from build123d import *

# Parameters (mm, degrees)
BOSS_EXTRUDE1_DEPTH                 = 170
CUT_EXTRUDE2_DEPTH                  = 1378.200029658
CUT_EXTRUDE2_DEPTH_BACK             = 1378.200029658
SKETCH7_W                           = 60.055026026
SKETCH7_H                           = 40
SKETCH7_H_2                         = 30
CUT_EXTRUDE7_DEPTH                  = 20.697901
FILLET1_R                           = 10
CUT_EXTRUDE3_REACH                  = 1001.772
CUT_EXTRUDE3_END_RADIUS             = 68.41639524
SKETCH3_R                           = 2.5
CUT_EXTRUDE3_DIRECTION_2_DEPTH      = 10
SKETCH4_R                           = 2.5
CUT_EXTRUDE4_DEPTH                  = 10
CUT_EXTRUDE4_DIRECTION_2_REACH      = 1377.394
CUT_EXTRUDE4_DIRECTION_2_END_RADIUS = 68.41639524
CUT_EXTRUDE5_REACH                  = 1377.394
SKETCH5_R                           = 5
CUT_EXTRUDE6_REACH                  = 1001.772
SKETCH6_R                           = 5


with BuildPart() as part:
    # Sketch1 → Boss-Extrude1 (new body)
    with BuildSketch(Plane.XY):
        with BuildLine():
            Line((1349.709167159, 7.051545827), (1340.728911037, -1.928710294))
            Line((1340.728911037, -1.928710294), (1340.375357647, -2.282263684))
            Line((1340.375357647, -2.282263684), (1361.562180969, -23.469087006))
            Line((1361.562180969, -23.469087006), (1354.491113157, -30.540154818))
            ThreePointArc((1354.491113157, -30.540154818), (1332.276376869, -15.701535719), (1306.072590331, -10.501468778))
            Line((1306.072590331, -10.501468778), (1306.072590331, -0.501468778))
            Line((1306.072590331, -0.501468778), (1336.035283217, -0.501468778))
            Line((1336.035283217, -0.501468778), (1336.035283217, -0.001468778))
            Line((1336.035283217, -0.001468778), (1336.072590331, 12.698531222))
            Line((1336.072590331, 12.698531222), (1336.072590331, 13.198531222))
            Line((1336.072590331, 13.198531222), (1321.072590331, 13.198531222))
            Line((1321.072590331, 13.198531222), (1321.072590331, 21.198531222))
            ThreePointArc((1321.072590331, 21.198531222), (1345.563373492, 16.327364444), (1366.326176516, 2.45535175))
            Line((1366.326176516, 2.45535175), (1360.669322267, -3.2015025))
            Line((1360.669322267, -3.2015025), (1350.062720549, 7.405099218))
            Line((1350.062720549, 7.405099218), (1349.709167159, 7.051545827))
        make_face()
    extrude(amount=-BOSS_EXTRUDE1_DEPTH)

    # Sketch2 → Cut-Extrude2 (cut, two sides: drawn at the far end of the back side and taken through both)
    with BuildSketch(Plane(origin=(0, 0, 0), x_dir=(1, 0, 0), z_dir=(0, 1, 0)).offset(-CUT_EXTRUDE2_DEPTH_BACK)):
        Polygon((1306.072590331, 165.353911181), (1366.326176516, 140.977580956), (1366.326176516, 170), (1306.072590331, 170), align=None)
        Polygon((1366.326176516, 4.246407684), (1353.192629401, 0), (1366.326176516, 0), align=None)
    extrude(amount=CUT_EXTRUDE2_DEPTH + CUT_EXTRUDE2_DEPTH_BACK, mode=Mode.SUBTRACT)

    # Sketch7 → Cut-Extrude7 (cut)
    with BuildSketch(Plane(origin=(187.283823237, 452.52498352, 0), x_dir=(-0.923993669874315, 0.38240776408461624, 0), z_dir=(-0.3824077640846163, -0.9239936698743151, 0))):
        with Locations((-1237.02208443, 145.353911181)):
            Rectangle(SKETCH7_W, SKETCH7_H)
        with Locations((-1237.02208443, 15)):
            Rectangle(SKETCH7_W, SKETCH7_H_2)
    extrude(amount=-CUT_EXTRUDE7_DEPTH, mode=Mode.SUBTRACT)

    # Fillet1
    fillet1_edges = [part.edges().sort_by_distance(p)[0] for p in [
        (1363.497749392, -0.373075375, -3.331905717),
        (1321.072590331, 17.198531222, 0),
        (1363.497749392, -0.373075375, -142.121855977),
        (1321.072590331, 17.198531222, -159.285476478),
        (1306.072590331, -5.501468778, -30),
        (1306.072590331, -5.501468778, -125.353911181),
        (1358.026647063, -27.004620912, -125.353911181),
        (1358.026647063, -27.004620912, -30),
    ]]
    fillet(fillet1_edges, radius=FILLET1_R)

    # Cut-Extrude3: up to this cylinder (the profile starts outside it)
    cut_extrude3_end = Plane(origin=(1306.113416139, -78.917851837, -77.676956), z_dir=(0, 0, 1)) * Cylinder(CUT_EXTRUDE3_END_RADIUS, 2201.37679048, mode=Mode.PRIVATE)
    # Sketch3 → Cut-Extrude3 (cut, up to the surface)
    with BuildSketch(Plane(origin=(661.975479169, 661.975479169, 0), x_dir=(0, 0, 1), z_dir=(0.7071067811866074, 0.7071067811864877, 0)), mode=Mode.PRIVATE) as cut_extrude3_sk1:
        with Locations(Location((-77.676955591, 971.365001741, 0), (0, 0, 270))):
            Circle(SKETCH3_R)
    cut_extrude3_tool1 = extrude(cut_extrude3_sk1.sketch, amount=-CUT_EXTRUDE3_REACH, mode=Mode.PRIVATE) - cut_extrude3_end
    add(cut_extrude3_tool1.solids().sort_by_distance((1348.834259, -24.883301, -77.676956))[0], mode=Mode.SUBTRACT)
    # Sketch3 → Cut-Extrude3 (cut, up to the surface)
    with BuildSketch(Plane(origin=(661.975479169, 661.975479169, 0), x_dir=(0, 0, 1), z_dir=(0.7071067811866074, 0.7071067811864877, 0)), mode=Mode.PRIVATE) as cut_extrude3_sk2:
        with Locations(Location((-107.676955591, 971.365001741, 0), (0, 0, 270))):
            Circle(SKETCH3_R)
    cut_extrude3_tool2 = extrude(cut_extrude3_sk2.sketch, amount=-CUT_EXTRUDE3_REACH, mode=Mode.PRIVATE) - cut_extrude3_end
    add(cut_extrude3_tool2.solids().sort_by_distance((1348.834259, -24.883301, -107.676956))[0], mode=Mode.SUBTRACT)
    # Sketch3 → Cut-Extrude3 (cut, up to the surface)
    with BuildSketch(Plane(origin=(661.975479169, 661.975479169, 0), x_dir=(0, 0, 1), z_dir=(0.7071067811866074, 0.7071067811864877, 0)), mode=Mode.PRIVATE) as cut_extrude3_sk3:
        with Locations(Location((-47.676955591, 971.365001741, 0), (0, 0, 270))):
            Circle(SKETCH3_R)
    cut_extrude3_tool3 = extrude(cut_extrude3_sk3.sketch, amount=-CUT_EXTRUDE3_REACH, mode=Mode.PRIVATE) - cut_extrude3_end
    add(cut_extrude3_tool3.solids().sort_by_distance((1348.834259, -24.883301, -47.676956))[0], mode=Mode.SUBTRACT)

    # Sketch3 → Cut-Extrude3 direction 2 (cut)
    with BuildSketch(Plane(origin=(661.975479169, 661.975479169, 0), x_dir=(0, 0, 1), z_dir=(0.7071067811866074, 0.7071067811864877, 0))):
        with Locations(Location((-77.676955591, 971.365001741, 0), (0, 0, 270))):
            Circle(SKETCH3_R)
        with Locations(Location((-107.676955591, 971.365001741, 0), (0, 0, 270))):
            Circle(SKETCH3_R)
        with Locations(Location((-47.676955591, 971.365001741, 0), (0, 0, 270))):
            Circle(SKETCH3_R)
    extrude(amount=CUT_EXTRUDE3_DIRECTION_2_DEPTH, mode=Mode.SUBTRACT)

    # Sketch4 → Cut-Extrude4 (cut)
    with BuildSketch(Plane(origin=(0, -10.501468778, 0), x_dir=(0, 0, 1), z_dir=(0, -1, 0))):
        with Locations((-107.676955591, -1314.072590331)):
            Circle(SKETCH4_R)
        with Locations((-77.676955591, -1314.072590331)):
            Circle(SKETCH4_R)
        with Locations((-47.676955591, -1314.072590331)):
            Circle(SKETCH4_R)
    extrude(amount=-CUT_EXTRUDE4_DEPTH, mode=Mode.SUBTRACT)

    # Cut-Extrude4 direction 2: up to this cylinder (the profile starts outside it)
    cut_extrude4_direction_2_end = Plane(origin=(1306.113416139, -78.917851837, -77.676956), z_dir=(0, 0, 1)) * Cylinder(CUT_EXTRUDE4_DIRECTION_2_END_RADIUS, 2952.62079048, mode=Mode.PRIVATE)
    # Sketch4 → Cut-Extrude4 direction 2 (cut, up to the surface)
    with BuildSketch(Plane(origin=(0, -10.501468778, 0), x_dir=(0, 0, 1), z_dir=(0, -1, 0)), mode=Mode.PRIVATE) as cut_extrude4_direction_2_sk1:
        with Locations((-107.676955591, -1314.072590331)):
            Circle(SKETCH4_R)
    cut_extrude4_direction_2_tool1 = extrude(cut_extrude4_direction_2_sk1.sketch, amount=CUT_EXTRUDE4_DIRECTION_2_REACH, mode=Mode.PRIVATE) - cut_extrude4_direction_2_end
    add(cut_extrude4_direction_2_tool1.solids().sort_by_distance((1314.07259, -10.501469, -107.676956))[0], mode=Mode.SUBTRACT)
    # Sketch4 → Cut-Extrude4 direction 2 (cut, up to the surface)
    with BuildSketch(Plane(origin=(0, -10.501468778, 0), x_dir=(0, 0, 1), z_dir=(0, -1, 0)), mode=Mode.PRIVATE) as cut_extrude4_direction_2_sk2:
        with Locations((-77.676955591, -1314.072590331)):
            Circle(SKETCH4_R)
    cut_extrude4_direction_2_tool2 = extrude(cut_extrude4_direction_2_sk2.sketch, amount=CUT_EXTRUDE4_DIRECTION_2_REACH, mode=Mode.PRIVATE) - cut_extrude4_direction_2_end
    add(cut_extrude4_direction_2_tool2.solids().sort_by_distance((1314.07259, -10.501469, -77.676956))[0], mode=Mode.SUBTRACT)
    # Sketch4 → Cut-Extrude4 direction 2 (cut, up to the surface)
    with BuildSketch(Plane(origin=(0, -10.501468778, 0), x_dir=(0, 0, 1), z_dir=(0, -1, 0)), mode=Mode.PRIVATE) as cut_extrude4_direction_2_sk3:
        with Locations((-47.676955591, -1314.072590331)):
            Circle(SKETCH4_R)
    cut_extrude4_direction_2_tool3 = extrude(cut_extrude4_direction_2_sk3.sketch, amount=CUT_EXTRUDE4_DIRECTION_2_REACH, mode=Mode.PRIVATE) - cut_extrude4_direction_2_end
    add(cut_extrude4_direction_2_tool3.solids().sort_by_distance((1314.07259, -10.501469, -47.676956))[0], mode=Mode.SUBTRACT)

    # Sketch5 → Cut-Extrude5 (cut, up to next)
    with BuildSketch(Plane(origin=(0, -10.501468778, 0), x_dir=(0, 0, 1), z_dir=(0, -1, 0)), mode=Mode.PRIVATE) as cut_extrude5_sk1:
        with Locations((-47.676955591, -1314.072590331)):
            Circle(SKETCH5_R)
    cut_extrude5_tool1 = extrude(cut_extrude5_sk1.sketch, amount=CUT_EXTRUDE5_REACH, mode=Mode.PRIVATE) & part.part
    # Sketch5 → Cut-Extrude5 (cut, up to next)
    with BuildSketch(Plane(origin=(0, -10.501468778, 0), x_dir=(0, 0, 1), z_dir=(0, -1, 0)), mode=Mode.PRIVATE) as cut_extrude5_sk2:
        with Locations((-77.676955591, -1314.072590331)):
            Circle(SKETCH5_R)
    cut_extrude5_tool2 = extrude(cut_extrude5_sk2.sketch, amount=CUT_EXTRUDE5_REACH, mode=Mode.PRIVATE) & part.part
    # Sketch5 → Cut-Extrude5 (cut, up to next)
    with BuildSketch(Plane(origin=(0, -10.501468778, 0), x_dir=(0, 0, 1), z_dir=(0, -1, 0)), mode=Mode.PRIVATE) as cut_extrude5_sk3:
        with Locations((-107.676955591, -1314.072590331)):
            Circle(SKETCH5_R)
    cut_extrude5_tool3 = extrude(cut_extrude5_sk3.sketch, amount=CUT_EXTRUDE5_REACH, mode=Mode.PRIVATE) & part.part
    add(cut_extrude5_tool1.solids().sort_by_distance((1314.07259, -10.501469, -47.676956))[0], mode=Mode.SUBTRACT)
    add(cut_extrude5_tool2.solids().sort_by_distance((1314.07259, -10.501469, -77.676956))[0], mode=Mode.SUBTRACT)
    add(cut_extrude5_tool3.solids().sort_by_distance((1314.07259, -10.501469, -107.676956))[0], mode=Mode.SUBTRACT)

    # Sketch6 → Cut-Extrude6 (cut, up to next)
    with BuildSketch(Plane(origin=(661.975479169, 661.975479169, 0), x_dir=(0, 0, 1), z_dir=(0.7071067811866074, 0.7071067811864877, 0)), mode=Mode.PRIVATE) as cut_extrude6_sk1:
        with Locations(Location((-107.676955591, 971.365001741, 0), (0, 0, 270))):
            Circle(SKETCH6_R)
    cut_extrude6_tool1 = extrude(cut_extrude6_sk1.sketch, amount=-CUT_EXTRUDE6_REACH, mode=Mode.PRIVATE) & part.part
    # Sketch6 → Cut-Extrude6 (cut, up to next)
    with BuildSketch(Plane(origin=(661.975479169, 661.975479169, 0), x_dir=(0, 0, 1), z_dir=(0.7071067811866074, 0.7071067811864877, 0)), mode=Mode.PRIVATE) as cut_extrude6_sk2:
        with Locations(Location((-77.676955591, 971.365001741, 0), (0, 0, 270))):
            Circle(SKETCH6_R)
    cut_extrude6_tool2 = extrude(cut_extrude6_sk2.sketch, amount=-CUT_EXTRUDE6_REACH, mode=Mode.PRIVATE) & part.part
    # Sketch6 → Cut-Extrude6 (cut, up to next)
    with BuildSketch(Plane(origin=(661.975479169, 661.975479169, 0), x_dir=(0, 0, 1), z_dir=(0.7071067811866074, 0.7071067811864877, 0)), mode=Mode.PRIVATE) as cut_extrude6_sk3:
        with Locations(Location((-47.676955591, 971.365001741, 0), (0, 0, 270))):
            Circle(SKETCH6_R)
    cut_extrude6_tool3 = extrude(cut_extrude6_sk3.sketch, amount=-CUT_EXTRUDE6_REACH, mode=Mode.PRIVATE) & part.part
    add(cut_extrude6_tool1.solids().sort_by_distance((1348.834259, -24.883301, -107.676956))[0], mode=Mode.SUBTRACT)
    add(cut_extrude6_tool2.solids().sort_by_distance((1348.834259, -24.883301, -77.676956))[0], mode=Mode.SUBTRACT)
    add(cut_extrude6_tool3.solids().sort_by_distance((1348.834259, -24.883301, -47.676956))[0], mode=Mode.SUBTRACT)


solid = part.part
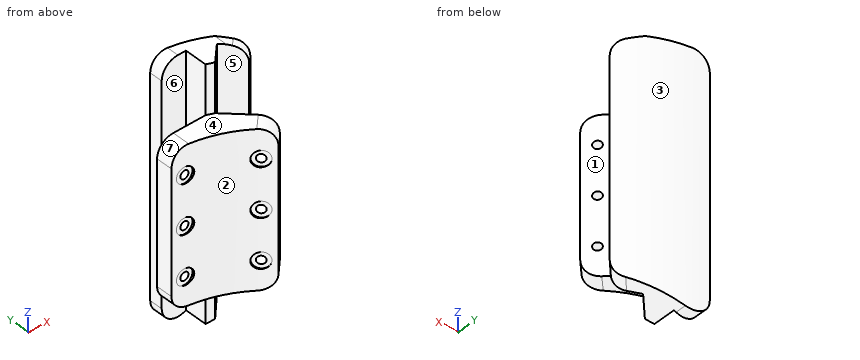
Can you work these out from the model? Positions are in its coordinate system, mm. Face numbers are marked on the shaded views. A direction names the side the tool comes from. Give positions to 0.01 mm unless a question says otherwise; leave off trailing zeros. Loops run counter-clockwise (first coordinate to the right, second up) from the corner with the lowest first, then second, coordinate; pieces in that order, holes last. Notation, with made-up numbers: (-35.75, 48) -> (-25.75, 48) arc R19 cw to (-25.75, 66) -> close; hole circle Ø7 at (-13, 44). An arc over 180 degrees is marked (long way). Write item = value, one per line.
1) Suppose I cut it at B-B on z = -86. Write out the boundary of the cut face in (x, y), then the cut area to 3 significant figures.
Check result:
outline = (1306.07, -10.5) arc R68.42 cw to (1354.49, -30.54) -> (1361.56, -23.47) -> (1340.38, -2.28) -> (1350.06, 7.41) -> (1360.67, -3.2) -> (1366.33, 2.46) arc R64 ccw to (1321.07, 21.2) -> (1321.07, 13.2) -> (1336.07, 13.2) -> (1336.07, 12.7) -> (1336.04, 0) -> (1336.04, -0.5) -> (1306.07, -0.5) -> close
area = 1,170 mm2
2) Suppose I cut it at C-C on y = 15.5. Write out the boundary of the cut face in (x, z).
Check result:
outline = (1321.07, -144.45) arc R10 ccw to (1334.82, -153.72) -> (1347.47, -148.61) -> (1347.47, 0) -> (1331.07, 0) arc R10 ccw to (1321.07, -10) -> close
3) I need wall thicknesses on L1, parallel to Z at x = 1313.5, y = -3.5; L2, parallel to Z at x = 1342.5, y = -18; L3, parallel to Z at x = 1345, y = -22. Which ranges of each line are inside material? Lowest first, please. Write a range as from..to.
Check result:
L1 = -125.02..-110.11, -105.24..-80.11, -75.24..-50.11, -45.24..-30.34
L2 = -125.35..-30
L3 = -125.35..-109.24, -106.12..-79.24, -76.12..-49.24, -46.12..-30
4) Will these pins go through, and if not, where does the flat tip stop? pin 1 (5 mm diameter, centred on y = 9, z = -120.5, fed in from +X); pin 2 (13 mm diameter, centred on x = 1314.07, z = -77.68, fed in from +Y); pin 3 (6 mm diameter, centred on y = 12, z = -102.5, fed in from +X); pin 4 (4.5 mm diameter, centred on x = 1314.07, z = -47.68, fed in from -Y).
Check result:
pin_1 = 1361.88
pin_2 = -0.5
pin_3 = 1358.66
pin_4 = through
5) Thinking about a two-plate mould opening in Y: for the marked faces 1, 2, 3 and 4, which applies, released by +Y, released by -Y, zero draft, split by the parting line, or undercut?
Check result:
face_1 = undercut
face_2 = released by -Y
face_3 = released by +Y
face_4 = zero draft
6) For the marked faces 5, 6 and 7, which set-ups out of +Z, -Z, +X, -X, +Y, -Y let a thin tool reach every point of the face, with its end or its side?
Check result:
face_5 = +Z, -Z
face_6 = +Z, -Z, -X
face_7 = +Z, -X, +Y, -Y
7) Suppose I cut it at A-A on x = 1328. Write out the boundary of the cut face in (y, z).
Check result:
outline = (-14.1, -125.35) -> (-0.5, -125.35) -> (-0.5, -30) -> (-14.1, -30) -> close; (13.2, -153.97) -> (20.82, -153.97) -> (20.82, -0.48) -> (13.2, -0.48) -> close
